Could you check a few things on this model? Use its own coordinates, in mm. Round coordinates to 2 decimals unless told otherwise and drop trailing zeros. Order: outer loops, then holes, each group sorted by start corner. A loop starts at its lowest first (then second) coordinate and runs counter-clockwise, first axis right, second up. Notation, with made-up numbers: (-29.5, -4) - (-0.5, -4) arc R25 ccw to (-0.5, 13) - close; hole circle Ø5 at (80.25, -12). An arc over 180 degrees is marked (long way). Use one line per item in the form item = value.
from build123d import *

# Parameters (mm, degrees)
F0_R     = 25
F1_DEPTH = 14
F1_TAPER = 20
F3_D     = 6.858
F4_R     = 0.762


with BuildPart() as f1:
    # F0 (on Top) → F1 (new body)
    with BuildSketch(Plane.XY):
        Circle(F0_R)
    extrude(amount=F1_DEPTH, taper=F1_TAPER)

    # F3 (through all)
    with Locations(Plane.XY.offset(14)):
        with Locations((0, 0)):
            Hole(F3_D / 2)

    # F4
    f4_edges = [f1.edges().sort_by_distance(p)[0] for p in [
        (-19.904417, 0, 14),
        (-25, 0, 0),
    ]]
    fillet(f4_edges, radius=F4_R)


solid = f1.part
Item 1: If we mould it in two halves opening along Y, with no side actions, what happens to faces 1 (the face through (5, 0, 0)), 2 (the face through (-16.115, -12.357, 12.893)), 3 (the face through (0.74, -3.35, 6.9))? For each: released by +Y, released by -Y, zero draft, split by the parting line, or undercut.
Found:
face_1 = zero draft
face_2 = split by the parting line
face_3 = undercut
Item 2: Will these pins go through, and if not, where does the flat tip stop? P1, Ø8, axis at x = -12, z = 9.5, coming from the -Y side; P2, Ø8, axis at x = 6, z = 9.5, coming from the +Y side; P3, Ø3, axis at y = 15, z = 2.5, coming from the +X side.
Found:
P1 = -20.63
P2 = 22.45
P3 = 20.15
Item 3: I need wall thicknesses on L1, parallel to Y at x = 7, z = 10.25; L2, parallel to Y at x = 0, z = 3.5; L3, parallel to Y at x = 0, z = 4.5. Which ranges of each line are inside material? Lowest first, please.
Found:
L1 = -20.08 to 20.08
L2 = -23.73 to -3.43, 3.43 to 23.73
L3 = -23.36 to -3.43, 3.43 to 23.36
Item 4: Imagine slicing it at A-A on x = 0. Please give me the cut outline in (y, z).
Found:
outline = (-24.63, 1.02) arc R0.76 ccw to (-23.91, 0) - (-3.43, 0) - (-3.43, 14) - (-19.37, 14) arc R0.76 ccw to (-20.09, 13.5) - close; (3.43, 0) - (23.91, 0) arc R0.76 ccw to (24.63, 1.02) - (20.09, 13.5) arc R0.76 ccw to (19.37, 14) - (3.43, 14) - close
Item 5: Imagine slicing it at C-C on z = 9.5. Please give me the cut outline in (x, y), plus the area to 3 significant figures.
Found:
outline = circle Ø43.08 at (0, 0); hole circle Ø6.86 at (0, 0)
area = 1,420 mm2
